Autodesk Inventor part; units mm, degrees
ref_plane "YZ Plane" through (0, 0, 0) normal (1, 0, 0) x (0, 1, 0)
ref_plane "XZ Plane" through (0, 0, 0) normal (0, 1, 0) x (-1, 0, 0)
ref_plane "XY Plane" through (0, 0, 0) normal (0, 0, 1) x (1, 0, 0)
sketch "Sketch1" plane through (0, 0, 0) normal (0, 1, 0) x (-1, 0, 0)
  line L0 (0, 0) -> (300, 0)
  line L1 (300, 0) -> (300, 300)
  line L2 (300, 300) -> (0, 300)
  line L3 (0, 300) -> (0, 0)
  dimension "d0" = 300
  dimension "d1" = 300
extrude "Extrusion1" add sketch "Sketch1" along normal blind 300
chamfer "Chamfer1" distance 100 distance2 300 1 edges at (-300, 150, 0) measured on face at (-100, 100, 0)
chamfer "Chamfer2" distance 100 distance2 300 1 edges at (-100, 0, 0) measured on face at (-66.6667, 100, 0)
chamfer "Chamfer3" distance 300 distance2 100 1 edges at (-100, 300, 0) measured on face at (-166.6667, 300, 200)
chamfer "Chamfer4" distance 150 distance2 200 1 edges at (-200.0001, 150, 0) measured on face at (-266.6667, 166.6667, 199.9999)
shell "Shell1" thickness 2 removed faces 1 at (-200, 100, 300)
properties part number "hopper"
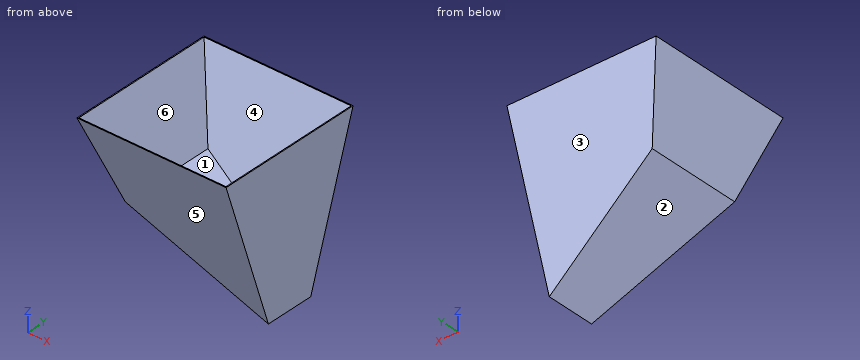
Can you work these out from the model? Positions are in its coordinate system, mm. Face numbers are marked on the shaded views. A direction names the side the tool comes from. Give positions to 0.01 mm unless a question says otherwise; leave off trailing zeros. Order: outer loops, then holes, each group sorted by start corner. A loop starts at its lowest first (then second) coordinate and runs counter-clockwise, first axis right, second up. Notation, with made-up numbers: M 54.25,57 L 68.25,57 A13 cw 68.25,66 Z; hole C 39.25,88 d4. An arc over 180 degrees is marked long. One line per question, with ' | ' between items.
Item 1: I'm going to push flat-ended pins straight in: pin 1 Ø12 at (x, y) = (-203, 209) entering from +Z; pin 2 Ø8 at (x, z) = (-91.5, 72.5) entering from +Y; pin 3 Ø12 at (x, y) = (-67.5, 143) entering from -Z. Where does each tip first touch, or does it pass through?
Answer block:
pin 1: stops at z = 122.51 | pin 2: stops at y = 225.5 | pin 3: stops at z = 35.37
Item 2: For the marked faces 5 and 6, which set-ups out of +Z, -Z, +X, -X, +Y, -Y let a thin tool reach every point of the face, with its end or its side?
Answer block:
face 5: -Z, +X, -X, -Y | face 6: +Z
Item 3: Suppose I cut it at B-B, the plane z = 153. Write out the boundary of the cut face in (x, y).
Answer block:
outline: M -251,49 L 0,49 L 0,251 L -251,251 Z; hole M -248.89,51.11 L -2,51.11 L -2,248.89 L -248.89,248.89 Z
Item 4: Suppose I cut it at D-D, the plane z = 41. Write out the boundary of the cut face in (x, y), then the cut area to 3 significant figures.
Answer block:
outline: M -71.29,86.33 L 0,86.33 L 0,213.67 L -71.29,213.67 Z; hole M -67.28,88.44 L -2,88.44 L -2,211.56 L -67.28,211.56 Z | area: 1,040 mm2
Item 5: We'd pull the mould along Y, two halves only. Please class the marked faces 1, 2, 3 and 4: released by +Y, released by -Y, zero draft, split by the parting line, or undercut.
Answer block:
face 1: undercut | face 2: zero draft | face 3: released by +Y | face 4: undercut
Item 6: Please list where these lines run through material, in increasing order: L1, parallel to Y at x = -49, z = 76.5; L2, parallel to X at y = 189.5, z = 90; L3, parallel to X at y = 225.5, z = 150.5.
Answer block:
L1: y = 74.5 to 76.61, 223.39 to 225.5 | L2: x = -156.49 to -152.48, -2 to 0 | L3: x = -250.17 to -248.06, -2 to 0
